Part print with two shaded views. Sizes in mm from the minimum x, y, z corner. Round coordinates to 2 decimals unless told otherwise and drop trailing zeros. Write each loop counter-clockwise with the first axis right and the second up, starting at its lowest first coordinate (ties: lowest second). Pieces come first, ordered by that corner, then holes. Notation, with made-up numbers: (-12.5, 52.25) -> (33.5, 52.25) arc R26 cw to (33.5, 84.25) -> close; hole circle Ø6 at (16, -1). An arc over 180 degrees is marked (long way). Put each result on its own line as item: value. Start each with the question number.
1. Saw through at D-D on y = 1.9. List the corners of the cut face in (x, z).
2. Drill centre lines: line 1 (X direction, y = 0.35, z = 15.9); line 2 (Y direction, x = 14.5, z = 19); line 3 (Z direction, x = 8.5, y = 0.5). Where is each one in solid material? Low to high. Write a range as from..to.
3. Saw through at B-B on x = 50. List the corners of the cut face in (y, z), and give its area (3 significant figures).
4. Pull direction Y, two halves, no side cores. Call the marked faces 1 and 2: pulls with the +Y half, pulls with the -Y half, needs draft (parallel to the pull), parting line crosses it, or undercut.
5. Saw through at A-A on x = 8.5. List the corners of the cut face in (y, z), and give its area (3 significant figures).
6. Flat gauge pins, fed straight in: P1, Ø12, axis at x = 34.5, z = 19, coming from the -Y side; P2, Ø12, axis at x = 34, z = 18, coming from the +Y side; P3, Ø1, axis at x = 27.5, y = 4.5, coming from the -Z side. Where does each tip first touch, or does it go through?
7. Saw through at C-C on x = 61.5. List the corners of the cut face in (y, z), and give its area (3 significant figures).
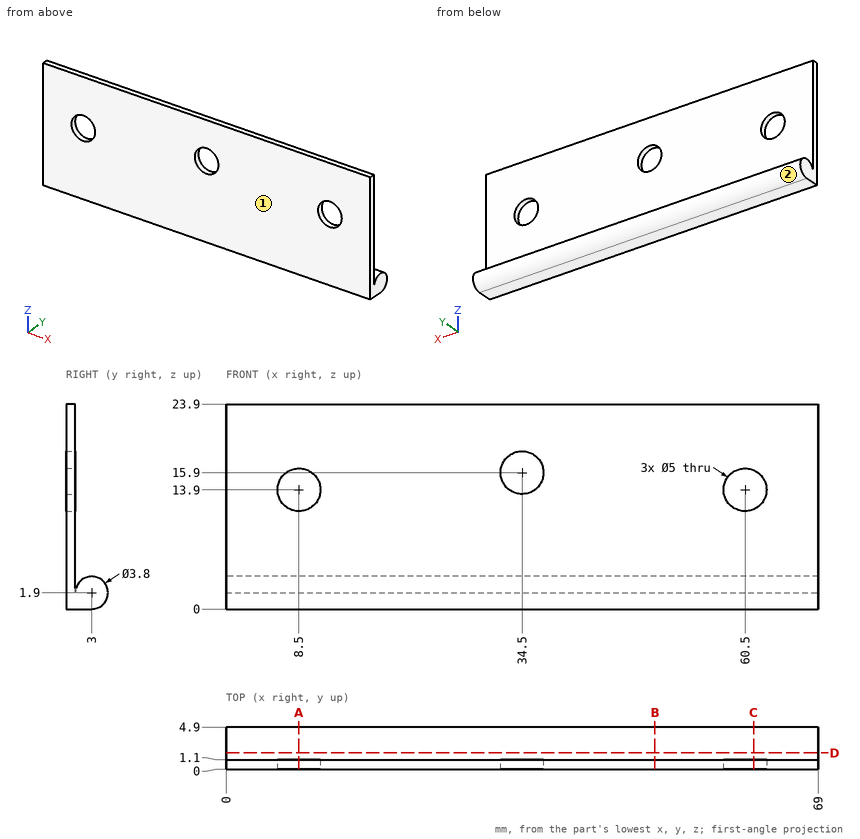
Return value:
1. outline: (0, 0) -> (69, 0) -> (69, 3.45) -> (0, 3.45) -> close
2. line 1: x = 0..7, 10..32, 37..59, 62..69
2. line 2: y = 0..1.1
2. line 3: z = 0..11.4, 16.4..23.9
3. outline: (0, 0) -> (3, 0) arc R1.9 ccw (long way) to (1.1, 1.9) -> (1.1, 23.9) -> (0, 23.9) -> close
3. area: 38.4 mm^2
4. face 1: pulls with the -Y half
4. face 2: undercut
5. outline: (0, 0) -> (3, 0) arc R1.9 ccw (long way) to (1.1, 1.9) -> (1.1, 11.4) -> (0, 11.4) -> close; (0, 16.4) -> (1.1, 16.4) -> (1.1, 23.9) -> (0, 23.9) -> close
5. area: 32.9 mm^2
6. P1: stops at y = 0
6. P2: stops at y = 1.1
6. P3: stops at z = 0.28
7. outline: (0, 0) -> (3, 0) arc R1.9 ccw (long way) to (1.1, 1.9) -> (1.1, 11.61) -> (0, 11.61) -> close; (0, 16.19) -> (1.1, 16.19) -> (1.1, 23.9) -> (0, 23.9) -> close
7. area: 33.4 mm^2
